from build123d import *

# Parameters (mm, degrees)
F1_DEPTH = 5.23875
F2_R     = 0.508
F3_DEPTH = 3.429
F5_D     = 1.778
F5_DEPTH = 3.302
F5_TIP   = 0.5341650903
F7_D     = 2.2606
F7_DEPTH = 3.429
F7_TIP   = 0.6791527577


with BuildPart() as f1:
    # F0 (on Top) → F1 (new body, symmetric)
    with BuildSketch(Plane.XY):
        Polygon((20.955, 28.575), (-20.955, -28.575), (20.955, -28.575), align=None)
        Polygon((-20.955, 28.575), (-20.955, -28.575), (20.955, 28.575), align=None)
    extrude(amount=F1_DEPTH, both=True)

    # F2 (on face) → F3 (cut)
    with BuildSketch(Plane(origin=(0, 28.575, 0), x_dir=(-1, 0, 0), z_dir=(0, 1, 0))):
        with Locations((-9.525, -1.75895)):
            Circle(F2_R)
        with Locations((9.525, -1.75895)):
            Circle(F2_R)
    extrude(amount=-F3_DEPTH, mode=Mode.SUBTRACT)

    # F5
    with Locations(Plane.YZ.offset(20.955)):
        with Locations((-18.415, -0.03175)):
            Hole(F5_D / 2, depth=F5_DEPTH)
            with Locations((0, 0, -(F5_DEPTH + F5_TIP / 2))):  # 118° drill point
                Cone(0, F5_D / 2, F5_TIP, mode=Mode.SUBTRACT)

    # F7
    with Locations(Plane.YZ.offset(20.955)):
        with Locations((-8.255, -0.03175)):
            Hole(F7_D / 2, depth=F7_DEPTH)
            with Locations((0, 0, -(F7_DEPTH + F7_TIP / 2))):  # 118° drill point
                Cone(0, F7_D / 2, F7_TIP, mode=Mode.SUBTRACT)


solid = f1.part
Could you check a few things on this model? Use its own coordinates, in mm. A direction names the side the tool comes from. Give positions to 0.01 mm unless a question says otherwise; leave off trailing zeros. Answer as CSV lines item,"result". Start each with the question number.
(1) I'm going to push a flat-ended pin straight in: pin 1 Ø0.8 at (x, z) = (9.52, -1.76) entering from +Y. Where does the tip first touch, or does it pass through?
(2) We'd pull the mould along Z, two halves only. Please class faces 1 (the flat face through (0, 0, -5.239)), 2 (the flat face through (0, -28.575, 0)), 3 (the conical face through (17, -8, 0)): released by +Z, released by -Z, zero draft, split by the parting line, or undercut.
(3) Which directions (+Z, -Z, +X, -X, +Y, -Y) give clear straight access to the entire face, cutting with the end or side of a thin tool? Please do faces 4 (the flat face through (-20.955, 0, 0)), 5 (the cylindrical face through (19.281, -19.236, -0.372)).
Computed:
1,pin 1,"stops at y = 25.15"
2,face 1,"released by -Z"
2,face 2,"zero draft"
2,face 3,"undercut"
3,face 4,"+Z, -Z, -X, +Y, -Y"
3,face 5,"+X"
